from build123d import *

# Parameters (mm, degrees)
F0_W     = 37.0614326914
F0_H     = 45.7304640924
F0_W_2   = 26.8021334539
F0_W_3   = 43.0278818478
F0_H_2   = 44.7304640924
F1_DEPTH = 20


with BuildPart() as f1:
    # F0 (on Top) → F1 (new body)
    with BuildSketch(Plane.XY):
        Polygon((73.9764403422, 1), (73.9764403422, 46.7304640924), (49.1905527413, 46.7304640924), (49.1905527413, 63.1642210121), (49.4113042951, 63.1642210121), (49.4113042951, 64.1642210121), (-53.0780255795, 64.1642210121), (-53.0780255795, 63.1642210121), (-53.0780255795, 46.7304640924), (-73.9764403422, 46.7304640924), (-73.9764403422, 1), (-79.9764403422, 1), (-79.9764403422, 0), (-73.9764403422, 0), (-73.9764403422, -46.7304640924), (73.9764403422, -46.7304640924), (73.9764403422, 0), (79.9764403422, 0), (79.9764403422, 1), align=None)
        with Locations((-54.4457239965, -22.8652320462)):
            Rectangle(F0_W, F0_H, mode=Mode.SUBTRACT)
        Polygon((-34.9150076509, 45.7304640924), (1.1464250405, 45.7304640924), (1.1464250405, 1), (1.1464250405, 0), (1.1464250405, -45.7304640924), (-34.9150076509, -45.7304640924), (-34.9150076509, 0), (-34.9150076509, 1), align=None, mode=Mode.SUBTRACT)
        with Locations((15.5474917675, -22.8652320462)):
            Rectangle(F0_W_2, F0_H, mode=Mode.SUBTRACT)
        with Locations((51.4624994183, -22.8652320462)):
            Rectangle(F0_W_3, F0_H, mode=Mode.SUBTRACT)
        Polygon((-72.9764403422, 1), (-72.9764403422, 45.7304640924), (-35.9150076509, 45.7304640924), (-35.9150076509, 1), (-52.0780255795, 1), (-52.0780255795, 23.0720378458), (-53.0780255795, 23.0720378458), (-53.0780255795, 1), align=None, mode=Mode.SUBTRACT)
        Polygon((-52.0780255795, 63.1642210121), (0, 63.1642210121), (1.1464250405, 46.7304640924), (-52.0780255795, 46.7304640924), align=None, mode=Mode.SUBTRACT)
        with Locations((15.5474917675, 23.3652320462)):
            Rectangle(F0_W_2, F0_H_2, mode=Mode.SUBTRACT)
        Polygon((29.9485584944, 1), (29.9485584944, 45.7304640924), (72.9764403422, 45.7304640924), (72.9764403422, 1), (49.1905527413, 1), (49.1905527413, 23.0720378458), (48.1905527413, 23.0720378458), (48.1905527413, 1), align=None, mode=Mode.SUBTRACT)
        Polygon((1, 63.1642210121), (48.1905527413, 63.1642210121), (48.1905527413, 46.7304640924), (2.1464250405, 46.7304640924), align=None, mode=Mode.SUBTRACT)
        Polygon((1.1464250405, 0), (1.1464250405, 1), (-34.9150076509, 1), (-34.9150076509, 0), (0, 0), align=None)
    extrude(amount=F1_DEPTH)


solid = f1.part
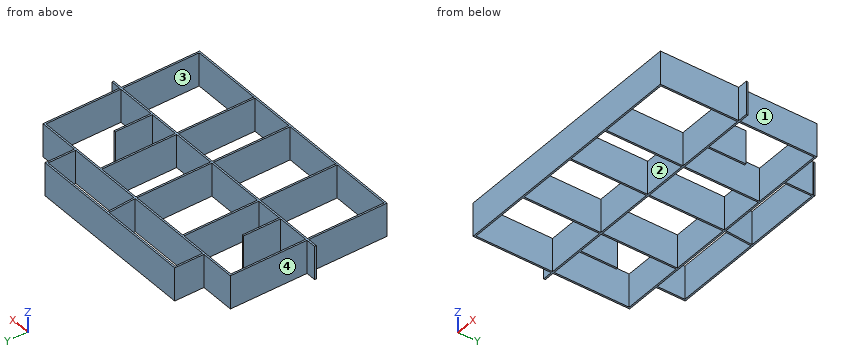
Geometry: final body of the model. Coordinates: model frame, mm. Face numbers are marked on the shaded views. A direction names the side the tool comes from. Coordinates: 2 decimals unless noted, no trailing zeros. Order: outer loops, then holes, each group sorted by start corner. A loop starts at its lowest first (then second) coordinate and runs counter-clockwise, first axis right, second up.
(1) Draft query along Y for the marked faces 1 and 2. Return one class per face: pulls with the +Y half, pulls with the -Y half, needs draft (parallel to the pull), parting line crosses it, or undercut.
(2) Material intervals for probe 1 along X at (y, z) = (47, 4); probe 2 along X at (y, z) = (45, 3.5) (3 decimals); probe 3 along Y at (x, z) = (48, 9.5), sorted ascending.
(3) Section query C-C (x = 16). Return the cut outline in (y, z).
(4) Section query B-B (y = 6). Return the cut outline in (x, z) (3 decimals), plus the area to 3 significant figures.
(5) Section query D-D (y = 43). Return the cut outline in (x, z) (3 decimals).
(6) First-contact query: pin 1 (10 mm diameter, centred on x = -40, y = 7, fed in from -Z); pin 2 (1 mm diameter, centred on y = 47.5, z = 9, fed in from +X); pin 3 (10 mm diameter, centred on y = 20.5, z = 15, fed in from -X); pin 4 (6 mm diameter, centred on x = -61.5, z = 12, fed in from +Y). Flat tips, straight axial feed; report the tip coordinate or a pass-through.
(7) Section query A-A (x = -68). Return the cut outline in (y, z).
(8) Access query for the marked faces 3 and 4. Directions: +Z, -Z, +X, -X, +Y, -Y. A direction counts if a zero-diameter tool reaches every point of the face in a straight line with its end or side. Return the directions, or none.
Solution:
1. face 1: needs draft
1. face 2: undercut
2. probe 1: x = -53.08 to -52.08, 1.13 to 2.13, 48.19 to 49.19
2. probe 2: x = -73.976 to -72.976, -35.915 to -34.915, 1.146 to 2.146, 28.949 to 29.949, 72.976 to 73.976
2. probe 3: y = -46.73 to -45.73, 0 to 1, 45.73 to 46.73, 63.16 to 64.16
3. outline: (-46.73, 0) - (-45.73, 0) - (-45.73, 20) - (-46.73, 20) - close; (0, 0) - (1, 0) - (1, 20) - (0, 20) - close; (45.73, 0) - (46.73, 0) - (46.73, 20) - (45.73, 20) - close; (63.16, 0) - (64.16, 0) - (64.16, 20) - (63.16, 20) - close
4. outline: (-73.976, 0) - (-72.976, 0) - (-72.976, 20) - (-73.976, 20) - close; (-53.078, 0) - (-52.078, 0) - (-52.078, 20) - (-53.078, 20) - close; (-35.915, 0) - (-34.915, 0) - (-34.915, 20) - (-35.915, 20) - close; (1.146, 0) - (2.146, 0) - (2.146, 20) - (1.146, 20) - close; (28.949, 0) - (29.949, 0) - (29.949, 20) - (28.949, 20) - close; (48.191, 0) - (49.191, 0) - (49.191, 20) - (48.191, 20) - close; (72.976, 0) - (73.976, 0) - (73.976, 20) - (72.976, 20) - close
4. area: 140 mm2
5. outline: (-73.976, 0) - (-72.976, 0) - (-72.976, 20) - (-73.976, 20) - close; (-35.915, 0) - (-34.915, 0) - (-34.915, 20) - (-35.915, 20) - close; (1.146, 0) - (2.146, 0) - (2.146, 20) - (1.146, 20) - close; (28.949, 0) - (29.949, 0) - (29.949, 20) - (28.949, 20) - close; (72.976, 0) - (73.976, 0) - (73.976, 20) - (72.976, 20) - close
6. pin 1: stops at z = 0
6. pin 2: stops at x = 49.19
6. pin 3: stops at x = -73.98
6. pin 4: stops at y = 46.73
7. outline: (-46.73, 0) - (-45.73, 0) - (-45.73, 20) - (-46.73, 20) - close; (0, 0) - (1, 0) - (1, 20) - (0, 20) - close; (45.73, 0) - (46.73, 0) - (46.73, 20) - (45.73, 20) - close
8. face 3: +Z, -Z
8. face 4: +Z, -Z, -X, +Y
